Could you check a few things on this model? Use its own coordinates, in mm. A direction names the side the tool comes from. Round coordinates to 2 decimals unless told otherwise and drop trailing zeros. Loops run counter-clockwise (first coordinate to the right, second up) from the corner with the lowest first, then second, coordinate; pieces in that order, holes last. Notation, with made-up numbers: M -29,-17 L 22,-17 A36 cw 22,21 Z; hole C -1,-33 d8. An arc over 180 degrees is marked long. One line per item, written item: value. Start each with the question number.
Q1. Imagine slicing it at A-A (z = 2.25). Please give me the cut outline in (x, y).
Q2. Imagine slicing it at D-D (x = -1.5). Please give me the cut outline in (y, z).
Q3. Imagine slicing it at C-C (z = 6). Please give me the cut outline in (x, y).
Q4. Please list where these lines run through material, in increasing order: line 1 along X through (y, z) = (0.2, 1.75); line 2 along X through (y, z) = (0.05, 3); line 3 along X through (y, z) = (0.3, 7.5).
Q5. Which directions (+Z, -Z, +X, -X, +Y, -Y) give clear straight access to the entire face, cutting with the end or side of a thin tool? Please do faces 4 (the face through (1.335, -0.006, 6.081)), 5 (the face through (-2, 0.4, 6)).
Q6. Imagine slicing it at B-B (y = 0). Please give me the cut outline in (x, z).
Q7. Thinking about a two-plate mould opening in X: for faces 1 (the face through (-1.36, -0.01, 6.06)), 2 (the face through (4.292, -0.006, 2.375)), 3 (the face through (-4.27, -0.01, 2.44)), which applies, released by +X, released by -X, zero draft, split by the parting line, or undercut?
from build123d import *

# Parameters (mm, degrees)
F1_DEPTH = 0.4


with BuildPart() as f1:
    # F0 (on Front) → F1 (new body, symmetric)
    with BuildSketch(Plane.XZ):
        with BuildLine():
            Line((-4.963131, 0.240064), (-4.2, 0))
            Line((-4.2, 0), (-2.837828, 4.33016))
            ThreePointArc((-2.837828, 4.33016), (-2.620056, 4.799444), (-2.289198, 5.197168))
            Line((-2.289198, 5.197168), (-0.407759, 6.94015))
            ThreePointArc((-0.407759, 6.94015), (-0.218986, 7.05861), (0, 7.1))
            ThreePointArc((0, 7.1), (0.218986, 7.05861), (0.407759, 6.94015))
            Line((0.407759, 6.94015), (2.289198, 5.197168))
            ThreePointArc((2.289198, 5.197168), (2.620056, 4.799444), (2.837828, 4.33016))
            Line((2.837828, 4.33016), (4.2, 0))
            Line((4.2, 0), (4.963131, 0.240064))
            Line((4.963131, 0.240064), (3.600959, 4.570224))
            ThreePointArc((3.600959, 4.570224), (3.296079, 5.227221), (2.832877, 5.784035))
            Line((2.832877, 5.784035), (0.951439, 7.527017))
            ThreePointArc((0.951439, 7.527017), (0.510968, 7.803423), (0, 7.9))
            ThreePointArc((0, 7.9), (-0.510968, 7.803423), (-0.951439, 7.527017))
            Line((-0.951439, 7.527017), (-2.832877, 5.784035))
            ThreePointArc((-2.832877, 5.784035), (-3.296079, 5.227221), (-3.600959, 4.570224))
            Line((-3.600959, 4.570224), (-4.963131, 0.240064))
        make_face()
    extrude(amount=F1_DEPTH, both=True)


solid = f1.part
Report:
1. outline: M -4.33,-0.4 L -3.49,-0.4 L -3.49,0.4 L -4.33,0.4 Z; M 3.49,-0.4 L 4.33,-0.4 L 4.33,0.4 L 3.49,0.4 Z
2. outline: M -0.4,5.93 L 0.4,5.93 L 0.4,7.02 L -0.4,7.02 Z
3. outline: M -2.6,-0.4 L -1.42,-0.4 L -1.42,0.4 L -2.6,0.4 Z; M 1.42,-0.4 L 2.6,-0.4 L 2.6,0.4 L 1.42,0.4 Z
4. line 1: x = -4.49 to -3.65, 3.65 to 4.49
4. line 2: x = -4.09 to -3.26, 3.26 to 4.09
4. line 3: x = -0.98 to 0.98
5. face 4: -Z, +Y, -Y
5. face 5: +Z, -Z, +X, -X, +Y
6. outline: M -4.96,0.24 L -4.2,0 L -2.84,4.33 A2 cw -2.29,5.2 L -0.41,6.94 A0.6 cw 0,7.1 A0.6 cw 0.41,6.94 L 2.29,5.2 A2 cw 2.84,4.33 L 4.2,0 L 4.96,0.24 L 3.6,4.57 A2.8 ccw 2.83,5.78 L 0.95,7.53 A1.4 ccw -0.95,7.53 L -2.83,5.78 A2.8 ccw -3.6,4.57 Z
7. face 1: undercut
7. face 2: released by +X
7. face 3: released by -X
